Work out the finished part from the listing and answer in its coordinate system (mm). A direction names the side the tool comes from. Give positions to 0.01 mm unless a question says otherwise; leave off trailing zeros. Write each loop counter-clockwise with the first axis right and the second up, starting at its lowest first coordinate (ties: lowest second). Pieces come first, ordered by that corner, then holes. Notation, with made-up numbers: (11.25, 10) -> (41.25, 10) arc R28 cw to (41.25, 43) -> close; hole circle Ø9 at (-24.5, -9.5). An arc over 180 degrees is marked (long way). Use a Markdown table: item, result. Add a question column.
Q1. Consider line 1 (X direction, y = 9.5, z = 1523.5); line 2 (Y direction, x = 1, z = 831). Determine where each line is inside the solid, lowest interval first.
Q2. For a pull along X with two mould halves and no side action, classify faces 1 (the face through (0, 19, 949)), 2 (the face through (36.512, 19, 949)), 3 (the face through (18, 1, 0)) as pulls with the +X half, pulls with the -X half, needs draft (parallel to the pull), parting line crosses it, or undercut.
Q3. Section C-C, the plane z = 1482.5 is taken. Give the vertices of the cut face in (x, y).
Q4. Section B-B, the plane x = 23 is taken. Give the vertices of the cut face in (y, z).
Q5. Section A-A, the plane y = 19.05 is taken. Give the vertices of the cut face in (x, z), plus the area to 3 significant figures.
Q6. For faces 4 (the face through (19, 38.1, 949)), 5 (the face through (1.588, 19, 949)), determine the directions among +Z, -Z, +X, -X, +Y, -Y from which every point of the face is accessible in a straight line to the end or side of a thin tool.
from build123d import *

# Parameters (mm, degrees)
SKETCH2_W                  = 38.1
SKETCH2_H                  = 38.1
SKETCH2_W_2                = 34.925
SKETCH2_H_2                = 34.925
BOSS_EXTRUDE1_DEPTH        = 1924.05
F_1_2_0_5_DIAMETER_HOLE1_D = 12.7


with BuildPart() as part:
    # Sketch2 → Boss-Extrude1 (new body)
    with BuildSketch(Plane.XY):
        with Locations((19.05, 19.05)):
            Rectangle(SKETCH2_W, SKETCH2_H)
        with Locations((19.05, 19.05)):
            Rectangle(SKETCH2_W_2, SKETCH2_H_2, mode=Mode.SUBTRACT)
    extrude(amount=BOSS_EXTRUDE1_DEPTH)

    # 1/2 (0.5) Diameter Hole1 (through all)
    with Locations(Plane.ZY):
        with Locations((831.85, 19.05)):
            Hole(F_1_2_0_5_DIAMETER_HOLE1_D / 2)


solid = part.part
Result set:
| question | item | result |
|---|---|---|
| 1 | line 1 | x = 0 to 1.59, 36.51 to 38.1 |
| 1 | line 2 | y = 0 to 12.76, 25.34 to 38.1 |
| 2 | face 1 | pulls with the -X half |
| 2 | face 2 | undercut |
| 2 | face 3 | needs draft |
| 3 | outline | (0, 0) -> (38.1, 0) -> (38.1, 38.1) -> (0, 38.1) -> close; hole (1.59, 1.59) -> (36.51, 1.59) -> (36.51, 36.51) -> (1.59, 36.51) -> close |
| 4 | outline | (0, 0) -> (1.59, 0) -> (1.59, 1924.05) -> (0, 1924.05) -> close; (36.51, 0) -> (38.1, 0) -> (38.1, 1924.05) -> (36.51, 1924.05) -> close |
| 5 | outline | (0, 0) -> (1.59, 0) -> (1.59, 825.5) -> (0, 825.5) -> close; (0, 838.2) -> (1.59, 838.2) -> (1.59, 1924.05) -> (0, 1924.05) -> close; (36.51, 0) -> (38.1, 0) -> (38.1, 825.5) -> (36.51, 825.5) -> close; (36.51, 838.2) -> (38.1, 838.2) -> (38.1, 1924.05) -> (36.51, 1924.05) -> close |
| 5 | area | 6,070 mm2 |
| 6 | face 4 | +Z, -Z, +X, -X, +Y |
| 6 | face 5 | +Z, -Z |
